from build123d import *

# Parameters (mm, degrees)
SKETCH1_W           = 85.09
SKETCH1_H           = 130.81
BOSS_EXTRUDE1_DEPTH = 186.69
SKETCH3_W           = 77.47
SKETCH3_H           = 38.1
CUT_EXTRUDE3_DEPTH  = 31.75
SKETCH4_W           = 179.07
SKETCH4_H           = 77.47
CUT_EXTRUDE4_DEPTH  = 127


with BuildPart() as part:
    # Sketch1 → Boss-Extrude1 (new body)
    with BuildSketch(Plane.YZ):
        with Locations((42.545, 65.405)):
            Rectangle(SKETCH1_W, SKETCH1_H)
    extrude(amount=BOSS_EXTRUDE1_DEPTH)

    # Sketch3 → Cut-Extrude3 (cut)
    with BuildSketch(Plane.YZ.offset(186.69)):
        with Locations((42.545, 111.76)):
            Rectangle(SKETCH3_W, SKETCH3_H)
    extrude(amount=-CUT_EXTRUDE3_DEPTH, mode=Mode.SUBTRACT)

    # Sketch4 → Cut-Extrude4 (cut)
    with BuildSketch(Plane(origin=(0, 0, 0), x_dir=(1, 0, 0), z_dir=(0, 0, -1))):
        with Locations((93.345, -42.545)):
            Rectangle(SKETCH4_W, SKETCH4_H)
    extrude(amount=-CUT_EXTRUDE4_DEPTH, mode=Mode.SUBTRACT)


solid = part.part
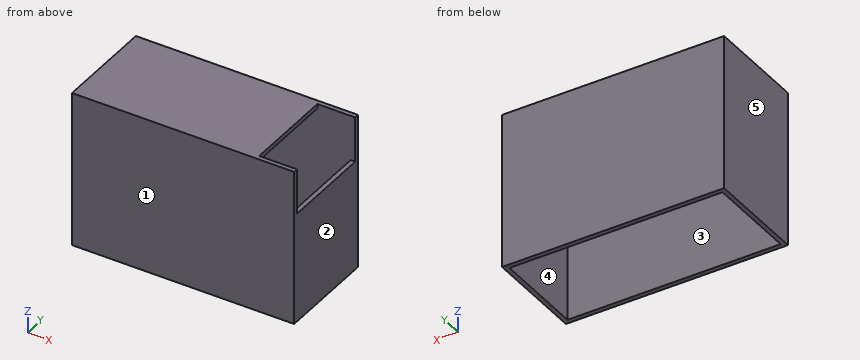
Input: part model. Units: mm. Frame: model coordinates. Face numbers are marked on the shaded views. A direction names the side the tool comes from. Coordinates: 2 decimals unless noted, no trailing zeros. Order: outer loops, then holes, each group sorted by start corner. A loop starts at its lowest first (then second) coordinate and runs counter-clockwise, first axis right, second up.
1. Access query for the marked faces 4 and 5. Directions: +Z, -Z, +X, -X, +Y, -Y. A direction counts if a zero-diameter tool reaches every point of the face in a straight line with its end or side. Return the directions, or none.
Checked values:
face 4: +Z, -Z
face 5: +Z, -Z, -X, +Y, -Y
2. Contact query for flat-ended pins moving along their axis: P1, Ø3, axis at y = 25.5, z = 128.5, coming from the +X side; P2, Ø1.9, axis at x = 185, y = 41.5, coming from the +Z side; P3, Ø23, axis at y = 51.5, z = 67.5, coming from the -X side; P4, Ø5, axis at y = 52, z = 96, coming from the +X side. Output: stop coordinate, or through.
Checked values:
P1: stops at x = 154.94
P2: stops at z = 92.71
P3: stops at x = 0
P4: stops at x = 3.81
3. Cut plane A-A, the plane x = 166.5. Return loops of the section in (y, z).
Checked values:
outline: (0, 0) - (3.81, 0) - (3.81, 130.81) - (0, 130.81) - close; (81.28, 0) - (85.09, 0) - (85.09, 130.81) - (81.28, 130.81) - close
4. Cut plane B-B, the plane z = 55.5. Return loops of the section in (x, y).
Checked values:
outline: (0, 0) - (186.69, 0) - (186.69, 85.09) - (0, 85.09) - close; hole (3.81, 3.81) - (182.88, 3.81) - (182.88, 81.28) - (3.81, 81.28) - close
5. Draft query along X for the marked faces 1, 2 and 3. Return one class per face: +X half, -X half, draft (parallel to the pull), parting line (faces both ways), or undercut.
Checked values:
face 1: draft
face 2: +X half
face 3: undercut
6. Cut plane D-D, the plane x = 88. Return loops of the section in (y, z), plus the area to 3 significant figures.
Checked values:
outline: (0, 0) - (3.81, 0) - (3.81, 127) - (81.28, 127) - (81.28, 0) - (85.09, 0) - (85.09, 130.81) - (0, 130.81) - close
area: 1,290 mm2
7. Ray query, line 1 along Y through (x, z) = (38.5, 90.5); line 2 along X through (y, z) = (39.5, 34.5); line 3 along Z through (x, y) = (121, 77.5). Return the intervals inside material, ascending.
Checked values:
line 1: y = 0 to 3.81, 81.28 to 85.09
line 2: x = 0 to 3.81, 182.88 to 186.69
line 3: z = 127 to 130.81
8. Cut plane C-C, the plane y = 18. Return loops of the section in (x, z), plus the area to 3 significant figures.
Checked values:
outline: (0, 0) - (3.81, 0) - (3.81, 127) - (154.94, 127) - (154.94, 130.81) - (0, 130.81) - close; (182.88, 0) - (186.69, 0) - (186.69, 92.71) - (182.88, 92.71) - close
area: 1,430 mm2
